from build123d import *

# Parameters (mm, degrees)
ESQUISSE1_R        = 1.75
BOSS_EXTRU_1_DEPTH = 2


with BuildPart() as part:
    # Esquisse1 → Boss.-Extru.1 (new body)
    with BuildSketch(Plane(origin=(0, 0, 0), x_dir=(1, 0, 0), z_dir=(0, 1, 0))):
        with BuildLine():
            Line((55.75, -70), (55.75, 15))
            Line((55.75, 15), (53.674026321, 40.47775659))
            ThreePointArc((53.674026321, 40.47775659), (51.771291303, 47.94288813), (47.510174455, 54.360946457))
            Line((47.510174455, 54.360946457), (40.217580929, 62.120740202))
            ThreePointArc((40.217580929, 62.120740202), (31.924250474, 67.945789429), (22, 70))
            Line((22, 70), (-22, 70))
            ThreePointArc((-22, 70), (-31.924250474, 67.945789429), (-40.217580929, 62.120740202))
            Line((-40.217580929, 62.120740202), (-47.510174455, 54.360946457))
            ThreePointArc((-47.510174455, 54.360946457), (-51.771291303, 47.94288813), (-53.674026321, 40.47775659))
            Line((-53.674026321, 40.47775659), (-55.75, 15))
            Line((-55.75, 15), (-55.75, -70))
            Line((-55.75, -70), (55.75, -70))
        make_face()
        with Locations(Location((-51.75, -66, 0), (0, 0, 270))):
            Circle(ESQUISSE1_R, mode=Mode.SUBTRACT)
        with Locations(Location((51.75, -66, 0), (0, 0, 270))):
            Circle(ESQUISSE1_R, mode=Mode.SUBTRACT)
        with Locations(Location((22, 66, 0), (0, 0, 270))):
            Circle(ESQUISSE1_R, mode=Mode.SUBTRACT)
        with Locations(Location((-22, 66, 0), (0, 0, 270))):
            Circle(ESQUISSE1_R, mode=Mode.SUBTRACT)
    extrude(amount=BOSS_EXTRU_1_DEPTH)


solid = part.part
Can you work these out from the model? Positions are in its coordinate system, mm. Give positions to 0.01 mm unless a question says otherwise; leave off trailing zeros. Loops run counter-clockwise (first coordinate to the right, second up) from the corner with the lowest first, then second, coordinate; pieces in that order, holes last. Notation, with made-up numbers: (77.5, 35.25) -> (101.5, 35.25) arc R22 cw to (101.5, 68.25) -> close; hole circle Ø1 at (22, 59). An arc over 180 degrees is marked (long way). Write item = value, one per line.
1) I need wall thicknesses on L1, parallel to X at y = 1.35, z = 66; L2, parallel to X at y = 0.45, z = -66; L3, parallel to Z at x = -20.5, y = 1.55. Which ranges of each line are inside material? Lowest first, please. Write a range as from..to.
Check result:
L1 = -55.75..-53.5, -50..50, 53.5..55.75
L2 = -35.56..-23.75, -20.25..20.25, 23.75..35.56
L3 = -70..-66.9, -65.1..70
2) Suppose I cut it at C-C on x = -51.75. Write out the boundary of the cut face in (y, z).
Check result:
outline = (0, -47.99) -> (2, -47.99) -> (2, 64.25) -> (0, 64.25) -> close; (0, 67.75) -> (2, 67.75) -> (2, 70) -> (0, 70) -> close
3) Suppose I cut it at B-B on z = 66. Write out the boundary of the cut face in (x, y).
Check result:
outline = (-55.75, 0) -> (-53.5, 0) -> (-53.5, 2) -> (-55.75, 2) -> close; (-50, 0) -> (50, 0) -> (50, 2) -> (-50, 2) -> close; (53.5, 0) -> (55.75, 0) -> (55.75, 2) -> (53.5, 2) -> close
4) Suppose I cut it at D-D on z = -66. Write out the boundary of the cut face in (x, y), then the cut area to 3 significant figures.
Check result:
outline = (-35.56, 0) -> (-23.75, 0) -> (-23.75, 2) -> (-35.56, 2) -> close; (-20.25, 0) -> (20.25, 0) -> (20.25, 2) -> (-20.25, 2) -> close; (23.75, 0) -> (35.56, 0) -> (35.56, 2) -> (23.75, 2) -> close
area = 128 mm2
5) Will this pin go through, and if not, where does the flat tip stop? pin 1 (5 mm diameter, centred on x = 6, z = 9, fed in from -Y).
Check result:
pin_1 = 0
6) Thinking about a two-plate mould opening in Z: for faces 1 (the cylindrical face through (-51.73, 0.99, -48.04)), 2 (the cylindrical face through (-52.42, 0.986, 67.617)), 3 (the flat face through (-1, 2, -1)), which applies, released by +Z, released by -Z, zero draft, split by the parting line, or undercut?
Check result:
face_1 = released by -Z
face_2 = undercut
face_3 = zero draft
7) Suppose I cut it at A-A on y = 0.4. Write out the boundary of the cut face in (x, z).
Check result:
outline = (-55.75, -15) -> (-53.67, -40.48) arc R23 ccw to (-47.51, -54.36) -> (-40.22, -62.12) arc R25 ccw to (-22, -70) -> (22, -70) arc R25 ccw to (40.22, -62.12) -> (47.51, -54.36) arc R23 ccw to (53.67, -40.48) -> (55.75, -15) -> (55.75, 70) -> (-55.75, 70) -> close; hole circle Ø3.5 at (-51.75, 66); hole circle Ø3.5 at (-22, -66); hole circle Ø3.5 at (22, -66); hole circle Ø3.5 at (51.75, 66)
